```python
from build123d import *

# Parameters (mm, degrees)
BOSS_EXTRUDE6_DEPTH = 1.3


with BuildPart() as part:
    # Sketch20 → Boss-Extrude6 (new body)
    with BuildSketch(Plane(origin=(0, 0, -30), x_dir=(-1, 0, 0), z_dir=(0, 1, 0))):
        with BuildLine():
            Line((1.53471655, 42.07642804), (0.605184619, 44.234777037))
            ThreePointArc((0.605184619, 44.234777037), (0, 47.17), (-0.605184619, 44.234777037))
            Line((-0.605184619, 44.234777037), (-1.53471655, 42.07642804))
            ThreePointArc((-1.53471655, 42.07642804), (-1.833529499, 42.220560049), (-2.118937454, 42.389691697))
            Line((-2.118937454, 42.389691697), (-3.377398231, 41.555494988))
            Line((-3.377398231, 41.555494988), (-3.730951621, 41.909048379))
            Line((-3.730951621, 41.909048379), (-4.084505012, 42.262601769))
            Line((-4.084505012, 42.262601769), (-3.250308303, 43.521062546))
            ThreePointArc((-3.250308303, 43.521062546), (-3.584652586, 44.155188282), (-3.796630085, 44.84))
            Line((-3.796630085, 44.84), (-5.276362383, 45.14))
            Line((-5.276362383, 45.14), (-5.276362383, 45.64))
            Line((-5.276362383, 45.64), (-5.276362383, 46.14))
            Line((-5.276362383, 46.14), (-3.796630085, 46.44))
            ThreePointArc((-3.796630085, 46.44), (-3.584652586, 47.124811718), (-3.250308303, 47.758937454))
            Line((-3.250308303, 47.758937454), (-4.084505012, 49.017398231))
            Line((-4.084505012, 49.017398231), (-3.730951621, 49.370951621))
            Line((-3.730951621, 49.370951621), (-3.377398231, 49.724505012))
            Line((-3.377398231, 49.724505012), (-2.118937454, 48.890308303))
            ThreePointArc((-2.118937454, 48.890308303), (-1.484811718, 49.224652586), (-0.8, 49.436630085))
            Line((-0.8, 49.436630085), (-0.5, 50.916362383))
            Line((-0.5, 50.916362383), (0, 50.916362383))
            Line((0, 50.916362383), (0.5, 50.916362383))
            Line((0.5, 50.916362383), (0.8, 49.436630085))
            ThreePointArc((0.8, 49.436630085), (1.484811718, 49.224652586), (2.118937454, 48.890308303))
            Line((2.118937454, 48.890308303), (3.377398231, 49.724505012))
            Line((3.377398231, 49.724505012), (3.730951621, 49.370951621))
            Line((3.730951621, 49.370951621), (4.084505012, 49.017398231))
            Line((4.084505012, 49.017398231), (3.250308303, 47.758937454))
            ThreePointArc((3.250308303, 47.758937454), (3.584652586, 47.124811718), (3.796630085, 46.44))
            Line((3.796630085, 46.44), (5.276362383, 46.14))
            Line((5.276362383, 46.14), (5.276362383, 45.64))
            Line((5.276362383, 45.64), (5.276362383, 45.14))
            Line((5.276362383, 45.14), (3.796630085, 44.84))
            ThreePointArc((3.796630085, 44.84), (3.584652586, 44.155188282), (3.250308303, 43.521062546))
            Line((3.250308303, 43.521062546), (4.084505012, 42.262601769))
            Line((4.084505012, 42.262601769), (3.730951621, 41.909048379))
            Line((3.730951621, 41.909048379), (3.377398231, 41.555494988))
            Line((3.377398231, 41.555494988), (2.118937454, 42.389691697))
            ThreePointArc((2.118937454, 42.389691697), (1.833529499, 42.220560049), (1.53471655, 42.07642804))
        make_face()
    extrude(amount=BOSS_EXTRUDE6_DEPTH)


solid = part.part
```
Geometry check sheet. Reference: the model listing, model coordinates, mm. A direction names the side the tool comes from. Round coordinates to 2 decimals unless told otherwise and drop trailing zeros. Order: outer loops, then holes, each group sorted by start corner. A loop starts at its lowest first (then second) coordinate and runs counter-clockwise, first axis right, second up. Notation, with made-up numbers: M -22.5,51 L 13.5,51 A22 ccw 13.5,77 Z; hole C 14,72.5 d6. An arc over 180 degrees is marked long. Answer as CSV lines item,"result".
1) Sectioned sample at B-B on x = 0. Record the cut outline in (y, z).
Entries:
outline,"M 0,17.17 L 1.3,17.17 L 1.3,20.92 L 0,20.92 Z"
2) Sectioned sample at D-D on z = 18.5. Record the cut outline in (x, y), and give its area (3 significant figures).
Entries:
outline,"M -3.74,0 L 3.74,0 L 3.74,1.3 L -3.74,1.3 Z"
area,"9.73 mm2"
3) Mould release check, pull along Z, two halves, no side actions. Record for faces 5 (the face through (-0.07, 1.3, 17.34)), 6 (the face through (-3.588, 0.641, 14.164)), 7 (the face through (-0.648, 0.641, 20.187)): +Z half, -Z half, draft (parallel to the pull), parting line (faces both ways), or undercut.
Entries:
face 5,"draft"
face 6,"undercut"
face 7,"+Z half"
4) Sectioned sample at C-C on z = 17. Record the cut outline in (x, y), and give its area (3 significant figures).
Entries:
outline,"M -3.63,0 L -0.7,0 L -0.7,1.3 L -3.63,1.3 Z; M 0.7,0 L 3.63,0 L 3.63,1.3 L 0.7,1.3 Z"
area,"7.63 mm2"
5) Thickness scan on probe 1 along X at (y, z) = (0.85, 15.64); probe 2 along Z at (x, y) = (0, 0.6); probe 3 along X at (y, z) = (0.8, 17). Record the ranges inside material, lowest first. Write a range as [from, to].
Entries:
probe 1,"[-5.28, -1.53], [1.53, 5.28]"
probe 2,"[17.17, 20.92]"
probe 3,"[-3.63, -0.7], [0.7, 3.63]"
6) Tool access check on faces 1 (the face through (3.673, 0.641, 12.883)), 2 (the face through (2.757, 0.641, 19.313)), 3 (the face through (-3.673, 0.641, 18.397)), 4 (the face through (-2.757, 0.641, 11.967)). Record the directions out of +Z, -Z, +X, -X, +Y, -Y that give a thin tool (end or side, any length) a straight path to the whole face; none if there is none.
Entries:
face 1,"+X, +Y, -Y"
face 2,"+Z, +Y, -Y"
face 3,"-X, +Y, -Y"
face 4,"-Z, +Y, -Y"
7) Sectioned sample at A-A on z = 15.64. Record the cut outline in (x, y).
Entries:
outline,"M -5.28,0 L -1.53,0 L -1.53,1.3 L -5.28,1.3 Z; M 1.53,0 L 5.28,0 L 5.28,1.3 L 1.53,1.3 Z"
8) Gauge pin test, flat end, axial feed: pin 1 Ø1.8 at (x, z) = (0, 15.64) entering from -Y. Record the tip position at first contact, or that the pin passes through.
Entries:
pin 1,"through"
